from build123d import *

# Parameters (mm, degrees)
SKETCH_R     = 8.95
SKETCH_W     = 8.2
SKETCH_H     = 8.2
PAD_DEPTH    = 4
SKETCH001_R  = 10.5
SKETCH001_W  = 8.2
SKETCH001_H  = 8.2
PAD001_DEPTH = 1


with BuildPart() as part:
    # Sketch → Pad (new body)
    with BuildSketch(Plane.XY):
        Circle(SKETCH_R)
        Rectangle(SKETCH_W, SKETCH_H, mode=Mode.SUBTRACT)
    extrude(amount=PAD_DEPTH)

    # Sketch001 → Pad001 (join)
    with BuildSketch(Plane.XY):
        Circle(SKETCH001_R)
        Rectangle(SKETCH001_W, SKETCH001_H, mode=Mode.SUBTRACT)
    extrude(amount=PAD001_DEPTH)


solid = part.part
The model under review builds one solid part; all positions refer to its coordinate system, in mm. A direction names the side the tool comes from. Round coordinates to 2 decimals unless told otherwise and drop trailing zeros. Loops run counter-clockwise (first coordinate to the right, second up) from the corner with the lowest first, then second, coordinate; pieces in that order, holes last. Notation, with made-up numbers: M 58,-22.75 L 104,-22.75 A22 cw 104,-7.75 Z; hole C 11.25,71 d9. An arc over 180 degrees is marked long. Answer as CSV lines item,"result". Start each with the question number.
Item 1: Consider section A-A (y = 0). Write out the cut boundary in (x, z), then the cut area to 3 significant figures.
Item 2: Wall thickness on line 1 (Z direction, x = 1, y = -9.5); line 2 (Y direction, x = 2.5, z = 3.6); line 3 (Y direction, x = 3.5, z = 1.05): over which ranges is each line inside the solid? List them lowest first. Write a range as [from, to].
Item 3: Consider section D-D (x = 7). Write out the cut boundary in (y, z), then the cut area to 3 significant figures.
Item 4: Mouldability with a two-part tool opening along Y and no side actions: class faces 1 (the face through (5, 0, 0)), 2 (the face through (-7.1, -5.45, 2.48)), 3 (the face through (0, -4.1, 2)) as released by +Y, released by -Y, zero draft, split by the parting line, or undercut.
Item 5: For faces 4 (the face through (8, 5, 1)), 5 (the face through (4.1, 0, 2)), list the 3-axis set-ups (+Z, -Z, +X, -X, +Y, -Y) from which the entire face can be reached by the end or side of a thin tool; tool diameter is ignored.
Item 6: Consider section C-C (z = 0.7). Write out the cut boundary in (x, y).
Item 7: Insertion check: P1, Ø1.5, axis at x = -4.5, z = 3, coming from the +Y side; P2, Ø1.2, axis at x = -2, z = 2, coming from the +Y side. Each pin has a flat end and moves straight along its axis. Give the tip position at first contact, or say it passes through.
Answer:
1,outline,"M -10.5,0 L -4.1,0 L -4.1,4 L -8.95,4 L -8.95,1 L -10.5,1 Z; M 4.1,0 L 10.5,0 L 10.5,1 L 8.95,1 L 8.95,4 L 4.1,4 Z"
1,area,"41.9 mm^2"
2,line 1,"z = [0, 1]"
2,line 2,"y = [-8.59, -4.1], [4.1, 8.59]"
2,line 3,"y = [-8.24, -4.1], [4.1, 8.24]"
3,outline,"M -7.83,0 L 7.83,0 L 7.83,1 L 5.58,1 L 5.58,4 L -5.58,4 L -5.58,1 L -7.83,1 Z"
3,area,"49.1 mm^2"
4,face 1,"zero draft"
4,face 2,"split by the parting line"
4,face 3,"undercut"
5,face 4,"+Z"
5,face 5,"+Z, -Z"
6,outline,"C 0,0 d21; hole M -4.1,-4.1 L 4.1,-4.1 L 4.1,4.1 L -4.1,4.1 Z"
7,P1,"stops at y = 8.13"
7,P2,"stops at y = 8.84"
